Could you check a few things on this model? Use its own coordinates, in mm. Give positions to 0.01 mm unless a question says otherwise; leave off trailing zeros. Write each loop counter-clockwise with the first axis right and the second up, starting at its lowest first coordinate (ties: lowest second). Pieces come first, ordered by that corner, then holes. Notation, with made-up numbers: (-31, 71.25) - (-11, 71.25) arc R28 ccw to (-11, 93.25) - close; hole circle Ø6 at (-28, -3.5). An arc over 180 degrees is marked (long way). Use one line per item in the form item = value.
```python
from build123d import *

# Parameters (mm, degrees)
SKETCH1_W           = 86
SKETCH1_H           = 86
SKETCH1_R           = 1.5
SKETCH1_R_2         = 1.75
SKETCH1_W_2         = 9
SKETCH1_H_2         = 24
SKETCH1_W_3         = 22
SKETCH1_H_3         = 60
BOSS_EXTRUDE1_DEPTH = 5
FILLET1_R           = 4


with BuildPart() as part:
    # Sketch1 → Boss-Extrude1 (new body)
    with BuildSketch(Plane.XY):
        with Locations((43, 43)):
            Rectangle(SKETCH1_W, SKETCH1_H)
        with Locations((25, 61)):
            Circle(SKETCH1_R, mode=Mode.SUBTRACT)
        with Locations((61, 61)):
            Circle(SKETCH1_R, mode=Mode.SUBTRACT)
        with Locations((61, 25)):
            Circle(SKETCH1_R, mode=Mode.SUBTRACT)
        with Locations((25, 25)):
            Circle(SKETCH1_R, mode=Mode.SUBTRACT)
        with Locations((25, 81)):
            Circle(SKETCH1_R, mode=Mode.SUBTRACT)
        with Locations(Location((25, 69, 0), (0, 0, 180))):
            Circle(SKETCH1_R, mode=Mode.SUBTRACT)
        with Locations((61, 69)):
            Circle(SKETCH1_R, mode=Mode.SUBTRACT)
        with Locations(Location((61, 81, 0), (0, 0, 180))):
            Circle(SKETCH1_R, mode=Mode.SUBTRACT)
        with Locations((64.920310217, 43)):
            Circle(SKETCH1_R_2, mode=Mode.SUBTRACT)
        with Locations((21.079689783, 43)):
            Circle(SKETCH1_R_2, mode=Mode.SUBTRACT)
        with Locations((75, 66)):
            Rectangle(SKETCH1_W_2, SKETCH1_H_2, mode=Mode.SUBTRACT)
        with BuildLine():
            Line((68.5, 61.5), (68.5, 60.5))
            ThreePointArc((68.5, 60.5), (67.5, 59.5), (66.5, 60.5))
            Line((66.5, 60.5), (66.5, 61.5))
            ThreePointArc((66.5, 61.5), (67.5, 62.5), (68.5, 61.5))
        make_face(mode=Mode.SUBTRACT)
        with BuildLine():
            Line((81.5, 61.5), (81.5, 60.5))
            ThreePointArc((81.5, 60.5), (82.5, 59.5), (83.5, 60.5))
            Line((83.5, 60.5), (83.5, 61.5))
            ThreePointArc((83.5, 61.5), (82.5, 62.5), (81.5, 61.5))
        make_face(mode=Mode.SUBTRACT)
        with BuildLine():
            Line((68.5, 24.5), (68.5, 25.5))
            ThreePointArc((68.5, 25.5), (67.5, 26.5), (66.5, 25.5))
            Line((66.5, 25.5), (66.5, 24.5))
            ThreePointArc((66.5, 24.5), (67.5, 23.5), (68.5, 24.5))
        make_face(mode=Mode.SUBTRACT)
        with BuildLine():
            Line((81.5, 24.5), (81.5, 25.5))
            ThreePointArc((81.5, 25.5), (82.5, 26.5), (83.5, 25.5))
            Line((83.5, 25.5), (83.5, 24.5))
            ThreePointArc((83.5, 24.5), (82.5, 23.5), (81.5, 24.5))
        make_face(mode=Mode.SUBTRACT)
        with Locations((75, 20)):
            Rectangle(SKETCH1_W_2, SKETCH1_H_2, mode=Mode.SUBTRACT)
        with BuildLine():
            Line((17.5, 61.5), (17.5, 60.5))
            ThreePointArc((17.5, 60.5), (18.5, 59.5), (19.5, 60.5))
            Line((19.5, 60.5), (19.5, 61.5))
            ThreePointArc((19.5, 61.5), (18.5, 62.5), (17.5, 61.5))
        make_face(mode=Mode.SUBTRACT)
        with BuildLine():
            Line((4.5, 61.5), (4.5, 60.5))
            ThreePointArc((4.5, 60.5), (3.5, 59.5), (2.5, 60.5))
            Line((2.5, 60.5), (2.5, 61.5))
            ThreePointArc((2.5, 61.5), (3.5, 62.5), (4.5, 61.5))
        make_face(mode=Mode.SUBTRACT)
        with BuildLine():
            Line((17.5, 24.5), (17.5, 25.5))
            ThreePointArc((17.5, 25.5), (18.5, 26.5), (19.5, 25.5))
            Line((19.5, 25.5), (19.5, 24.5))
            ThreePointArc((19.5, 24.5), (18.5, 23.5), (17.5, 24.5))
        make_face(mode=Mode.SUBTRACT)
        with BuildLine():
            Line((4.5, 24.5), (4.5, 25.5))
            ThreePointArc((4.5, 25.5), (3.5, 26.5), (2.5, 25.5))
            Line((2.5, 25.5), (2.5, 24.5))
            ThreePointArc((2.5, 24.5), (3.5, 23.5), (4.5, 24.5))
        make_face(mode=Mode.SUBTRACT)
        with Locations((11, 20)):
            Rectangle(SKETCH1_W_2, SKETCH1_H_2, mode=Mode.SUBTRACT)
        with Locations((11, 66)):
            Rectangle(SKETCH1_W_2, SKETCH1_H_2, mode=Mode.SUBTRACT)
        with Locations((43, 43)):
            Rectangle(SKETCH1_W_3, SKETCH1_H_3, mode=Mode.SUBTRACT)
        with BuildLine():
            Line((68.5, 70.5), (68.5, 71.5))
            ThreePointArc((68.5, 71.5), (67.5, 72.5), (66.5, 71.5))
            Line((66.5, 71.5), (66.5, 70.5))
            ThreePointArc((66.5, 70.5), (67.5, 69.5), (68.5, 70.5))
        make_face(mode=Mode.SUBTRACT)
        with BuildLine():
            Line((81.5, 70.5), (81.5, 71.5))
            ThreePointArc((81.5, 71.5), (82.5, 72.5), (83.5, 71.5))
            Line((83.5, 71.5), (83.5, 70.5))
            ThreePointArc((83.5, 70.5), (82.5, 69.5), (81.5, 70.5))
        make_face(mode=Mode.SUBTRACT)
        with BuildLine():
            Line((17.5, 70.5), (17.5, 71.5))
            ThreePointArc((17.5, 71.5), (18.5, 72.5), (19.5, 71.5))
            Line((19.5, 71.5), (19.5, 70.5))
            ThreePointArc((19.5, 70.5), (18.5, 69.5), (17.5, 70.5))
        make_face(mode=Mode.SUBTRACT)
        with BuildLine():
            Line((4.5, 70.5), (4.5, 71.5))
            ThreePointArc((4.5, 71.5), (3.5, 72.5), (2.5, 71.5))
            Line((2.5, 71.5), (2.5, 70.5))
            ThreePointArc((2.5, 70.5), (3.5, 69.5), (4.5, 70.5))
        make_face(mode=Mode.SUBTRACT)
        with BuildLine():
            Line((4.5, 15.5), (4.5, 14.5))
            ThreePointArc((4.5, 14.5), (3.5, 13.5), (2.5, 14.5))
            Line((2.5, 14.5), (2.5, 15.5))
            ThreePointArc((2.5, 15.5), (3.5, 16.5), (4.5, 15.5))
        make_face(mode=Mode.SUBTRACT)
        with BuildLine():
            Line((17.5, 15.5), (17.5, 14.5))
            ThreePointArc((17.5, 14.5), (18.5, 13.5), (19.5, 14.5))
            Line((19.5, 14.5), (19.5, 15.5))
            ThreePointArc((19.5, 15.5), (18.5, 16.5), (17.5, 15.5))
        make_face(mode=Mode.SUBTRACT)
        with BuildLine():
            Line((68.5, 15.5), (68.5, 14.5))
            ThreePointArc((68.5, 14.5), (67.5, 13.5), (66.5, 14.5))
            Line((66.5, 14.5), (66.5, 15.5))
            ThreePointArc((66.5, 15.5), (67.5, 16.5), (68.5, 15.5))
        make_face(mode=Mode.SUBTRACT)
        with BuildLine():
            Line((81.5, 15.5), (81.5, 14.5))
            ThreePointArc((81.5, 14.5), (82.5, 13.5), (83.5, 14.5))
            Line((83.5, 14.5), (83.5, 15.5))
            ThreePointArc((83.5, 15.5), (82.5, 16.5), (81.5, 15.5))
        make_face(mode=Mode.SUBTRACT)
    extrude(amount=BOSS_EXTRUDE1_DEPTH)

    # Fillet1
    fillet1_edges = [part.edges().sort_by_distance(p)[0] for p in [
        (32, 73, 2.5),
        (32, 13, 2.5),
        (54, 13, 2.5),
        (54, 73, 2.5),
        (0, 86, 2.5),
        (86, 86, 2.5),
        (86, 0, 2.5),
        (0, 0, 2.5),
    ]]
    fillet(fillet1_edges, radius=FILLET1_R)


solid = part.part
```
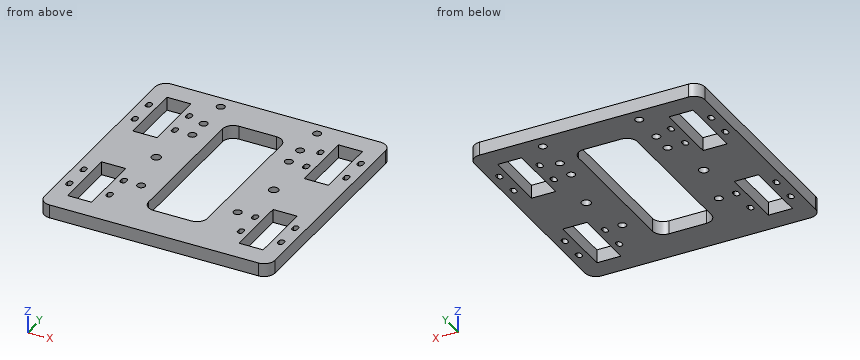
1. If I drill on line 1 (Y direction, x = 25, z = 2.7); line 2 (X direction, y = 69, z = 2.85); line 3 (Y direction, x = 10.5, z = 2.9), over which ranges is the centre line in solid material (lowest first)? Write a range as from..to.
Response values:
line_1 = 0..23.5, 26.5..59.5, 62.5..67.5, 70.5..79.5, 82.5..86
line_2 = 0..6.5, 15.5..23.5, 26.5..32, 54..59.5, 62.5..70.5, 79.5..86
line_3 = 0..8, 32..54, 78..86
2. Imagine slicing it at C-C, the plane y = 43. List the corners of the cut face in (x, z) for me.
Response values:
outline = (0, 0) - (19.33, 0) - (19.33, 5) - (0, 5) - close; (22.83, 0) - (32, 0) - (32, 5) - (22.83, 5) - close; (54, 0) - (63.17, 0) - (63.17, 5) - (54, 5) - close; (66.67, 0) - (86, 0) - (86, 5) - (66.67, 5) - close
3. Imagine slicing it at D-D, the plane x = 40. List the corners of the cut face in (y, z) for me, and give its area (3 significant figures).
Response values:
outline = (0, 0) - (13, 0) - (13, 5) - (0, 5) - close; (73, 0) - (86, 0) - (86, 5) - (73, 5) - close
area = 130 mm²
4. Imagine slicing it at A-A, the plane y = 34. List the corners of the cut face in (x, z) for me.
Response values:
outline = (0, 0) - (32, 0) - (32, 5) - (0, 5) - close; (54, 0) - (86, 0) - (86, 5) - (54, 5) - close
5. Imagine slicing it at B-B, the plane x = 25. List the corners of the cut face in (y, z) for me, and give its area (3 significant figures).
Response values:
outline = (0, 0) - (23.5, 0) - (23.5, 5) - (0, 5) - close; (26.5, 0) - (59.5, 0) - (59.5, 5) - (26.5, 5) - close; (62.5, 0) - (67.5, 0) - (67.5, 5) - (62.5, 5) - close; (70.5, 0) - (79.5, 0) - (79.5, 5) - (70.5, 5) - close; (82.5, 0) - (86, 0) - (86, 5) - (82.5, 5) - close
area = 370 mm²
